Verification items for the finished model (mm, model axes). Face numbers are marked on the shaded views. A direction names the side the tool comes from. Give positions to 0.01 mm unless a question says otherwise; leave off trailing zeros. Write each loop counter-clockwise with the first axis right and the second up, starting at its lowest first coordinate (ties: lowest second). Pieces come first, ordered by that corner, then holes. Notation, with made-up numbers: (-19, -24.5) - (36, -24.5) arc R24 cw to (36, 7.5) - close; hole circle Ø5 at (3.25, -28.75). An arc over 180 degrees is marked (long way). Answer as a JSON object with one key per item and string values. Group by question number.
Item 1: Draft check along X on the marked faces 1, 2 and 3. Enter one of: +X half, -X half, draft (parallel to the pull), parting line (faces both ways), or undercut.
Item 2: Go/stop test with flat-tipped pins: pin 1 (1.9 mm diameter, centred on y = -17.5, z = 9.5, fed in from +X); pin 2 (3 mm diameter, centred on x = -11.5, y = -2, fed in from -Z); pin 3 (0.6 mm diameter, centred on x = -19.5, z = 4, fed in from -Y). Record where each tip stops, or that it passes through.
Item 3: Tool access check on the marked faces 4, 5, 6 and 7. Record the directions out of +Z, -Z, +X, -X, +Y, -Y that give a thin tool (end or side, any length) a straight path to the whole face; none if there is none.
Item 4: Scan lines: line 1 along Y through (x, z) = (8, 9.75); line 2 along Y through (x, z) = (-15.5, 0.3). Record each from-to range of solid material in increasing order. Write a range as [from, to].
Item 5: Sectioned sample at D-D, the plane x = 10. Record the boundary of the cut face in (y, z).
Item 6: Sectioned sample at B-B, the plane x = 16.5. Record the boundary of the cut face in (y, z), and give its area (3 significant figures).
Item 7: Sectioned sample at A-A, the plane z = 5.5. Count the separate pieces of the cut face and the enclosed holes in it, and give its area (3 significant figures).
```python
from build123d import *

# Parameters (mm, degrees)
PAD_DEPTH              = 12
POCKET_DEPTH           = 11
POCKET001_DEPTH        = 11
POLARPATTERN_COUNT     = 4
SKETCH003_R            = 1.6
POCKET002_DEPTH        = 127.655658
POLARPATTERN001_COUNT  = 4
SKETCH004_W            = 4
SKETCH004_H            = 20
POCKET003_DEPTH        = 12.001
SKETCH005_W            = 15
SKETCH005_H            = 7
POCKET004_DEPTH        = 40.001
SKETCH006_W            = 1.5
SKETCH006_H            = 8
POCKET005_DEPTH        = 40.001
LINEARPATTERN_COUNT    = 6
LINEARPATTERN_PITCH    = 3.6
SKETCH007_W            = 1.5
SKETCH007_H            = 19
POCKET006_DEPTH        = 12.001
LINEARPATTERN001_COUNT = 8
LINEARPATTERN001_PITCH = 3.714286


with BuildPart() as part:
    # Sketch → Pad (new body)
    with BuildSketch(Plane.XY):
        with BuildLine():
            Line((-15, 20), (15, 20))
            ThreePointArc((20, 15), (18.535534, 18.535534), (15, 20))
            Line((20, 15), (20, -15))
            ThreePointArc((15, -20), (18.535534, -18.535534), (20, -15))
            Line((15, -20), (-15, -20))
            ThreePointArc((-20, -15), (-18.535534, -18.535534), (-15, -20))
            Line((-20, -15), (-20, 15))
            ThreePointArc((-15, 20), (-18.535534, 18.535534), (-20, 15))
        make_face()
    extrude(amount=PAD_DEPTH)

    # Sketch001 (on Face9 of Pad) → Pocket (cut)
    with BuildSketch(Plane(origin=(0, 0, 0), x_dir=(1, 0, 0), z_dir=(0, 0, -1))):
        with BuildLine():
            ThreePointArc((-15.5, 11), (-12.318019, 12.318019), (-11, 15.5))
            Line((-11, 15.5), (-11, 19.3))
            Line((-11, 19.3), (11, 19.3))
            Line((11, 19.3), (11, 15.5))
            ThreePointArc((11, 15.5), (12.318019, 12.318019), (15.5, 11))
            Line((15.5, 11), (19.3, 11))
            Line((19.3, 11), (19.3, -11))
            Line((19.3, -11), (15.5, -11))
            ThreePointArc((15.5, -11), (12.318019, -12.318019), (11, -15.5))
            Line((11, -15.5), (11, -19.3))
            Line((-11, -19.3), (11, -19.3))
            Line((-11, -15.5), (-11, -19.3))
            ThreePointArc((-11, -15.5), (-12.318019, -12.318019), (-15.5, -11))
            Line((-19.3, -11), (-15.5, -11))
            Line((-19.3, 11), (-19.3, -11))
            Line((-19.3, 11), (-15.5, 11))
        make_face()
    extrude(amount=-POCKET_DEPTH, mode=Mode.SUBTRACT)

    # Sketch002 (on Face5 of Pocket) → Pocket001 (cut)
    with BuildSketch(Plane.XY.offset(12)):
        with BuildLine():
            ThreePointArc((-15.5, 11.9), (-12.954416, 12.954416), (-11.9, 15.5))
            Line((-11.9, 20.654364), (-11.9, 15.5))
            Line((-20.945524, 20.654364), (-11.9, 20.654364))
            Line((-20.945524, 11.9), (-20.945524, 20.654364))
            Line((-15.5, 11.9), (-20.945524, 11.9))
        make_face()
    pocket001 = extrude(amount=-POCKET001_DEPTH, mode=Mode.SUBTRACT)

    # PolarPattern: Pocket001 ×4 about axis
    polarpattern_axis = Axis((0, 0, 12), (0, 0, 1))
    for i in range(1, POLARPATTERN_COUNT):
        add(pocket001.rotate(polarpattern_axis, i * 360 / POLARPATTERN_COUNT), mode=Mode.SUBTRACT)

    # Sketch003 (on Face2 of PolarPattern) → Pocket002 (cut, through all)
    with BuildSketch(Plane(origin=(0, 0, 0), x_dir=(1, 0, 0), z_dir=(0, 0, -1))):
        with Locations((-15.5, 15.5)):
            Circle(SKETCH003_R)
    pocket002 = extrude(amount=-POCKET002_DEPTH, mode=Mode.SUBTRACT)

    # PolarPattern001: Pocket002 ×4 about axis
    polarpattern001_axis = Axis((0, 0, 0), (0, 0, -1))
    for i in range(1, POLARPATTERN001_COUNT):
        add(pocket002.rotate(polarpattern001_axis, i * 360 / POLARPATTERN001_COUNT), mode=Mode.SUBTRACT)

    # Sketch004 (on Face6 of PolarPattern001) → Pocket003 (cut, through all)
    with BuildSketch(Plane.XY.offset(12)):
        with Locations((16.7, 0)):
            Rectangle(SKETCH004_W, SKETCH004_H)
    extrude(amount=-POCKET003_DEPTH, mode=Mode.SUBTRACT)

    # Sketch005 (on Face10 of Pocket003) → Pocket004 (cut, through all)
    with BuildSketch(Plane.XZ.offset(20)):
        with Locations((-3.689, 3.5)):
            Rectangle(SKETCH005_W, SKETCH005_H)
    extrude(amount=-POCKET004_DEPTH, mode=Mode.SUBTRACT)

    # Sketch006 (on Face31 of Pocket004) → Pocket005 (cut, through all)
    with BuildSketch(Plane.YZ.offset(20)):
        with Locations((-9.225517, 5.5)):
            Rectangle(SKETCH006_W, SKETCH006_H)
    pocket005 = extrude(amount=-POCKET005_DEPTH, mode=Mode.SUBTRACT)

    # LinearPattern: Pocket005 ×6
    with Locations(*[(0, i * LINEARPATTERN_PITCH, 0) for i in range(1, LINEARPATTERN_COUNT)]):
        add(pocket005, mode=Mode.SUBTRACT)

    # Sketch007 (on Face9 of LinearPattern) → Pocket006 (cut, through all)
    with BuildSketch(Plane.XY.offset(12)):
        with Locations((-14.75, 0)):
            Rectangle(SKETCH007_W, SKETCH007_H)
    pocket006 = extrude(amount=-POCKET006_DEPTH, mode=Mode.SUBTRACT)

    # LinearPattern001: Pocket006 ×8
    with Locations(*[(i * LINEARPATTERN001_PITCH, 0, 0) for i in range(1, LINEARPATTERN001_COUNT)]):
        add(pocket006, mode=Mode.SUBTRACT)


solid = part.part
```
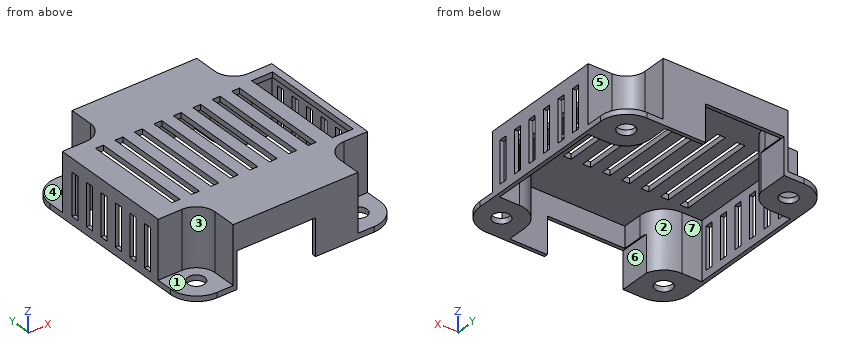
Geometry check:
{
 "1": {"face 1": "draft", "face 2": "undercut", "face 3": "-X half"},
 "2": {"pin 1": "x = 11.9", "pin 2": "z = 11", "pin 3": "y = -11.9"},
 "3": {"face 4": "+Z, -X, +Y", "face 5": "+Z, +X, +Y", "face 6": "-Z, +Y, -Y", "face 7": "-Z"},
 "4": {"line 1": "[-20, -19.3], [19.3, 20]", "line 2": "[-19.97, -17.1], [-13.9, -11], [11, 13.9], [17.1, 19.97]"},
 "5": {"outline": "(-20, 0) - (-19.3, 0) - (-19.3, 11) - (19.3, 11) - (19.3, 0) - (20, 0) - (20, 12) - (-20, 12) - close"},
 "6": {"outline": "(-19.77, 0) - (-16.75, 0) - (-16.75, 1) - (-19.77, 1) - close; (-14.25, 0) - (-11, 0) - (-11, 11) - (-10, 11) - (-10, 12) - (-11.9, 12) - (-11.9, 1) - (-14.25, 1) - close; (10, 11) - (11, 11) - (11, 0) - (14.25, 0) - (14.25, 1) - (11.9, 1) - (11.9, 12) - (10, 12) - close; (16.75, 0) - (19.77, 0) - (19.77, 1) - (16.75, 1) - close", "area": "34.3 mm^2"},
 "7": {"separate pieces": "14", "enclosed holes": "0", "area": "81.5 mm^2"}
}
